from build123d import *

# Parameters (mm, degrees)
SKETCH1_R           = 1.4605
BOSS_EXTRUDE1_DEPTH = 2.54
SKETCH12_W          = 3.175
SKETCH12_H          = 17.78
BOSS_EXTRUDE7_DEPTH = 2.54
FILLET6_R           = 19.05
FILLET7_R           = 6.35
FILLET8_R           = 3.175
FILLET9_R           = 2.2225
CHAMFER1_SIZE       = 1.27
CHAMFER1_SIZE2      = 1.226424744
FILLET10_R          = 2.2225


with BuildPart() as part:
    # Sketch1 → Boss-Extrude1 (new body)
    with BuildSketch(Plane(origin=(0, 0, 0), x_dir=(1, 0, 0), z_dir=(0, 1, 0))):
        Polygon((0, 0), (69.85, 0), (69.85, -21.59), (50.8, -21.59), (38.1, -38.1), (34.192307692, -43.18), (0, -43.18), (0, -38.1), align=None)
        with Locations(Location((41.275, -15.24, 0), (0, 0, 270))):
            Circle(SKETCH1_R, mode=Mode.SUBTRACT)
    extrude(amount=BOSS_EXTRUDE1_DEPTH)

    # Sketch12 → Boss-Extrude7 (add)
    with BuildSketch(Plane.XZ):
        with Locations((66.3575, 10.795)):
            Rectangle(SKETCH12_W, SKETCH12_H)
    extrude(amount=BOSS_EXTRUDE7_DEPTH)

    # Fillet6
    fillet6_edges = [part.edges().sort_by_distance(p)[0] for p in [
        (50.8, 1.27, 21.59),
    ]]
    fillet(fillet6_edges, radius=FILLET6_R)

    # Fillet7
    fillet7_edges = [part.edges().sort_by_distance(p)[0] for p in [
        (34.192307692, 1.27, 43.18),
        (0, 1.27, 43.18),
    ]]
    fillet(fillet7_edges, radius=FILLET7_R)

    # Fillet8
    fillet8_edges = [part.edges().sort_by_distance(p)[0] for p in [
        (69.85, 1.27, 0),
        (69.85, 1.27, 21.59),
    ]]
    fillet(fillet8_edges, radius=FILLET8_R)

    # Fillet9
    fillet9_edges = [part.edges().sort_by_distance(p)[0] for p in [
        (0, 1.27, 0),
    ]]
    fillet(fillet9_edges, radius=FILLET9_R)

    # Chamfer1
    chamfer1_edges = [part.edges().sort_by_distance(p)[0] for p in [
        (41.275, 2.54, 13.7795),
    ]]
    chamfer1_side = [part.faces().sort_by_distance(p)[0] for p in [
        (29.97778843, 2.54, 18.654075923),
    ]]
    chamfer(chamfer1_edges, length=CHAMFER1_SIZE, length2=CHAMFER1_SIZE2, reference=chamfer1_side[0])

    # Fillet10
    fillet10_edges = [part.edges().sort_by_distance(p)[0] for p in [
        (63.427624263, 2.54, 21.59),
        (51.764877453, 2.54, 23.549533953),
        (18.707779092, 2.54, 43.18),
        (40.589741024, 2.54, 34.863336669),
        (33.870681875, 2.54, 42.526822016),
        (1.859871939, 2.54, 41.320128061),
        (34.44875, 2.54, 0),
        (69.85, 2.54, 10.795),
        (68.92006403, 2.54, 20.66006403),
        (68.92006403, 2.54, 0.92993597),
        (0, 2.54, 19.52625),
        (0.650955179, 2.54, 0.650955179),
    ]]
    fillet(fillet10_edges, radius=FILLET10_R)


solid = part.part
Verification items for the finished model (mm, model axes). A direction names the side the tool comes from. Coordinates: 2 decimals unless noted, no trailing zeros. Loops run counter-clockwise (first coordinate to the right, second up) from the corner with the lowest first, then second, coordinate; pieces in that order, holes last. Notation, with made-up numbers: (71, -21) -> (101, -21) arc R16 cw to (101, 0) -> close; hole circle Ø1 at (31, 37). An arc over 180 degrees is marked (long way). Write each question's results on one line, items separated by ' | '.
Item 1: Mould release check, pull along Z, two halves, no side actions. Record for faces 1 (the face through (0.67, 0.16, 0.63)), 2 (the face through (67.945, -1, 11)), 3 (the face through (51.87, 0.16, 23.5)), 4 (the face through (39.979, 0.648, 15.914)): +Z half, -Z half, draft (parallel to the pull), parting line (faces both ways), or undercut.
Found:
face 1: -Z half | face 2: draft | face 3: +Z half | face 4: undercut
Item 2: Material ranges on L1, parallel to X at y = 0.55, z = 15.24; L2, parallel to Y at x = 38, z = 34; L3, parallel to X at y = 1, z = 15.24, recorded low to high.
Found:
L1: x = 0.01 to 39.81, 42.74 to 69.84 | L2: y = 0 to 2.54 | L3: x = 0.11 to 39.81, 42.74 to 69.74
Item 3: Tool access check on faces 5 (the face through (66, -1, 1.905)), 6 (the face through (63.38, 1.91, 20.92)), 7 (the face through (18.53, 1.91, 42.51)), 8 (the face through (64.77, -1, 11)), 9 (the face through (0.67, 1.91, 19.28)). Record the directions out of +Z, -Z, +X, -X, +Y, -Y that give a thin tool (end or side, any length) a straight path to the whole face; none if there is none.
Found:
face 5: -Z, +X, -X, -Y | face 6: +Z, +X, +Y | face 7: +Z, +X, -X, +Y | face 8: +Z, -Z, -X, -Y | face 9: +Z, -Z, -X, +Y
Item 4: Gauge pin test, flat ends, axial feed: pin 1 (21.5 mm diameter, centred on x = 37, z = 25.5, fed in from -Y); pin 2 (10 mm diameter, centred on x = 46, z = 37.5, fed in from +Y); pin 3 (2 mm diameter, centred on x = 38, y = 1, fed in from +Z); pin 4 (1.5 mm diameter, centred on y = 2, z = 24, fed in from +X). Record the tip position at first contact, or that the pin passes through.
Found:
pin 1: stops at y = 0 | pin 2: passes through | pin 3: stops at z = 39.42 | pin 4: stops at x = 51.23
Item 5: Section check D-D, the plane y = -0.7. Enter the section's corners in (x, z) (3 decimals).
Found:
outline: (64.77, 1.905) -> (67.945, 1.905) -> (67.945, 19.685) -> (64.77, 19.685) -> close
